Autodesk Inventor part; units mm, degrees
ref_plane "Plano de trabalho1" through (0, 28, 0) normal (0, 1, 0) x (-1, 0, 0)
ref_plane "YZ Plane" through (0, 0, 0) normal (1, 0, 0) x (0, 1, 0)
ref_plane "XY Plane" through (0, 0, 0) normal (0, 0, 1) x (1, 0, 0)
sketch "Esboço1" plane through (0, 0, 0) normal (0, 0, 1) x (1, 0, 0)
  circle A0 centre (0, 0) radius 18.75
  dimension "d2" = 37.5
extrude "Extrusão1" add sketch "Esboço1" along normal blind 28.9
sketch "Esboço2" plane through (0, 0, 28.9) normal (0, 0, 1) x (1, 0, 0)
  circle A0 centre (0, 0) radius 28
  dimension "d3" = 56
extrude "Extrusão2" add sketch "Esboço2" along normal blind 89.8
sketch "Esboço3" plane through (0, 0, 118.7) normal (0, 0, 1) x (1, 0, 0)
  circle A0 centre (0, 0) radius 43.6
  dimension "d6" = 87.2
extrude "Extrusão3" add sketch "Esboço3" along normal blind 24
sketch "Esboço4" plane through (0, 0, 142.7) normal (0, 0, 1) x (1, 0, 0)
  circle A0 centre (0, 0) radius 28
  dimension "d9" = 56
extrude "Extrusão4" add sketch "Esboço4" along normal blind 247.1
ref_plane "Plano de trabalho1" through (0, 28, 0) normal (0, 1, 0) x (-1, 0, 0)
sketch "Esboço5" plane through (0, 28, 0) normal (0, 1, 0) x (-1, 0, 0)
  line L0 (86.1192, 180.9) -> (-95.7284, 180.9)
  line L1 (-95.7284, 180.9) -> (-95.7284, 374.7)
  line L2 (-95.7284, 374.7) -> (86.1192, 374.7)
  line L3 (86.1192, 374.7) -> (86.1192, 180.9)
  line L4 (43.6, 142.7) -> (-43.6, 142.7)
  point P0 (0, 0)
  dimension "d13" = 193.8
  dimension "d14" = 38.2
extrude "Extrusão5" cut sketch "Esboço5" against normal blind 29
sketch "Esboço6" plane through (0, -1, 0) normal (0, 1, 0) x (1, 0, 0)
  circle A0 centre (0, -227.8) radius 6.25
  circle A1 centre (0, -327.8) radius 6.25
  line L0 (28, -180.9) -> (-28, -180.9)
  line L1 (-28, -374.7) -> (28, -374.7)
  point P0 (0, 0)
  point P1 (-27.9821, -180.9)
  point P2 (27.9821, -180.9)
  point P3 (27.9821, -374.7)
  point P4 (-27.9821, -374.7)
  dimension "d17" = 12.5
  dimension "d19" = 100
  dimension "d20" = 12.5
  dimension "d21" = 46.9
extrude "Extrusão6" cut sketch "Esboço6" against normal up to next
chamfer "Chanfro1" distance 1 angle 45 1 edges at (-18.75, 0, 0)
properties part number "eixo da Valvula"
Input: part model. Units: mm. Frame: model coordinates. A direction names the side the tool comes from. Give positions to 0.01 mm unless a question says otherwise; leave off trailing zeros. Write each loop counter-clockwise with the first axis right and the second up, starting at its lowest first coordinate (ties: lowest second). Pieces come first, ordered by that corner, then holes. Notation, with made-up numbers: M 43,51 L 55,51 A23 cw 55,63 Z; hole C 13,53.5 d2. An arc over 180 degrees is marked long. Write item = value, one per line. Start each with the question number.
1) Cut plane A-A on x = 0. Count the separate pieces of the cut face and the enclosed holes in it, then the cut area to 3 significant figures.
2) Material intervals for line 1 along Z through (x, y) = (0, -22.25); line 2 along Z through (x, y) = (0, -7); line 3 along Z through (x, y) = (-24.5, -4), sorted ascending. Write a range as [from, to].
3) Cut plane D-D on x = 34.5. Return the cut outline in (y, z).
4) Cut plane C-C on z = 128.5. Return the cut outline in (x, y), then the cut area to 3 significant figures.
5) Cut plane B-B on z = 227.8. Return the cut outline in (x, y), then the cut area to 3 significant figures.
6) Draft query along X for faces 1 (the flat face through (-0.6, -28.5, 142.7)), 2 (the cylindrical face through (3.36, -14.31, 322.53)), 3 (the cylindrical face through (-2.44, -18.59, 14.75)), 4 (the cylindrical face through (2.884, -14.311, 233.345)). Return one class per face: +X half, -X half, draft (parallel to the pull), parting line (faces both ways), or undercut.
7) Reachability of faces 5 (the flat face through (6, -18, 28.9)), 6 (the flat face through (0, 10, 374.7)), 7 (the flat face through (0, 0, 389.8)) from +Z, -Z, +X, -X, +Y, -Y: full face, straight path, thin tool, end or side. Return the list, or none.
8) First-contact query: pin 1 Ø1 at (x, y) = (15.5, -20) entering from -Z; pin 2 Ø3 at (y, z) = (-31, 279.5) entering from -X; pin 3 Ø10 at (x, z) = (-9, 58) entering from +Y; pin 4 Ø23 at (x, y) = (-5, 12.5) entering from -Z. Flat tips, straight axial feed; report the tip coordinate or a pass-through.
Solved:
q1.separate_pieces = 3
q1.enclosed_holes = 0
q1.area = 15,700 mm2
q2.line_1 = [28.9, 221.55], [234.05, 321.55], [334.05, 389.8]
q2.line_2 = [0, 221.55], [234.05, 321.55], [334.05, 389.8]
q2.line_3 = [28.9, 389.8]
q3.outline = M -26.66,118.7 L 26.66,118.7 L 26.66,142.7 L -26.66,142.7 Z
q4.outline = C 0,0 d87.2
q4.area = 5,970 mm2
q5.outline = M -27.98,-1 A28 ccw -6.25,-27.29 L -6.25,-1 Z; M 6.25,-27.29 A28 ccw 27.98,-1 L 6.25,-1 Z
q5.area = 841 mm2
q6.face_1 = draft
q6.face_2 = undercut
q6.face_3 = parting line
q6.face_4 = undercut
q7.face_5 = -Z
q7.face_6 = +X, -X, +Y
q7.face_7 = +Z, +X, -X, +Y, -Y
q8.pin_1 = 28.9
q8.pin_2 = through
q8.pin_3 = 27.71
q8.pin_4 = 0
